Here's the drawing with two shaded views (mm, measured from the low corner). I have some questions. A direction names the side the tool comes from. Round coordinates to 2 decimals unless told otherwise and drop trailing zeros. Loops run counter-clockwise (first coordinate to the right, second up) from the corner with the lowest first, then second, coordinate; pieces in that order, holes last.
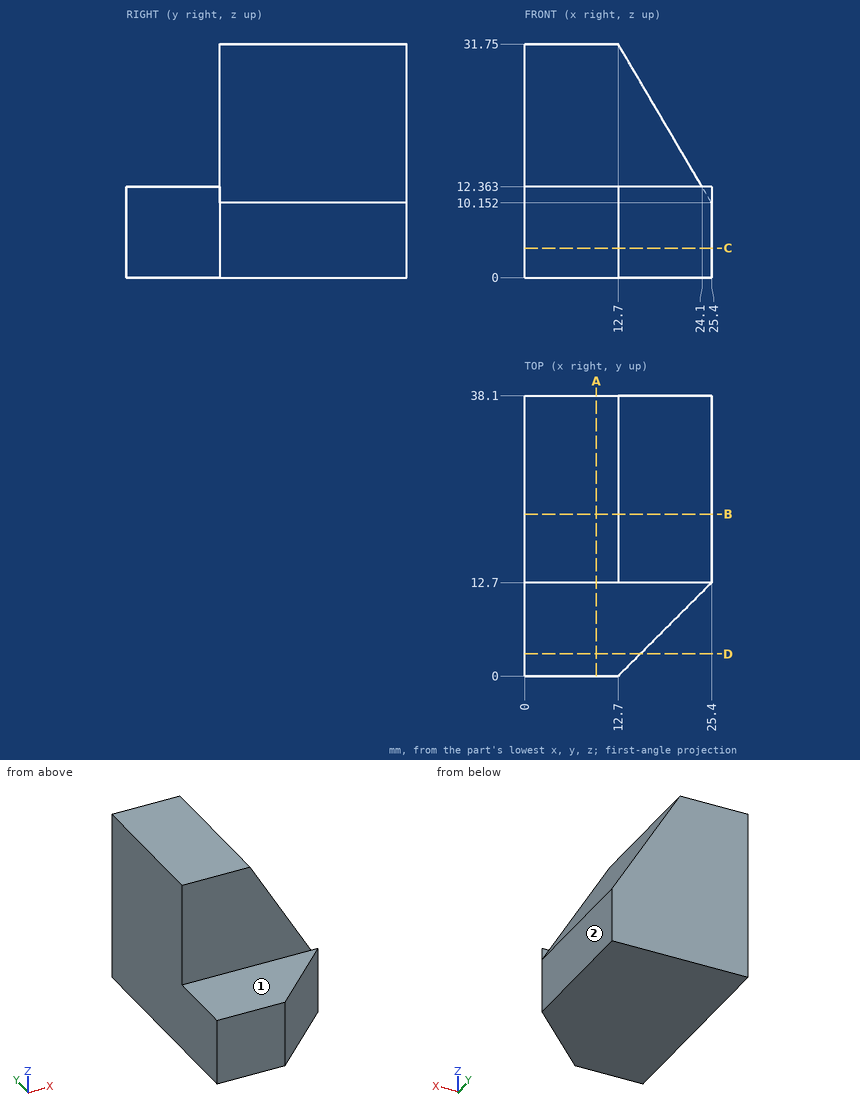
(1) If we section it at D-D, the plane y = 3: List the corners of the cut face in (x, z) for me.
Worked answers:
outline: (0, 0) - (15.7, 0) - (15.7, 12.36) - (0, 12.36) - close
(2) Will these pins go through, and if not, where does the flat tip stop? P1, Ø1.5, axis at x = 14.5, y = 27, coming from the +Z side (1 decimal); P2, Ø6, axis at x = 11.5, z = 18, coming from the -Y side.
Worked answers:
P1: stops at z = 30
P2: stops at y = 12.7
(3) If we section it at C-C, the plane z = 4: List the corners of the cut face in (x, y) for me, then the cut area to 3 significant figures.
Worked answers:
outline: (0, 0) - (12.7, 0) - (25.4, 12.7) - (25.4, 38.1) - (0, 38.1) - close
area: 887 mm2
(4) For the marked faces 1 and 2, which set-ups out of +Z, -Z, +X, -X, +Y, -Y let a thin tool reach every point of the face, with its end or its side?
Worked answers:
face 1: +Z, +X, -X, -Y
face 2: +Z, -Z, +X, +Y, -Y
(5) If I drill on line 1 (Z direction, x = 9, y = 8.5); line 2 (Y direction, x = 20.5, z = 15); line 3 (X direction, y = 3, z = 5), over which ranges is the centre line in solid material (lowest first)?
Worked answers:
line 1: z = 0 to 12.36
line 2: y = 12.7 to 38.1
line 3: x = 0 to 15.7
(6) If we section it at A-A, the plane x = 9.75: List the corners of the cut face in (y, z) for me.
Worked answers:
outline: (0, 0) - (38.1, 0) - (38.1, 31.75) - (12.7, 31.75) - (12.7, 12.36) - (0, 12.36) - close
(7) If we section it at B-B, the plane y = 22: List the corners of the cut face in (x, z) for me.
Worked answers:
outline: (0, 0) - (25.4, 0) - (25.4, 10.15) - (12.7, 31.75) - (0, 31.75) - close
